```python
from build123d import *

# Parameters (mm, degrees)
F0_W     = 72.2630545497
F0_H     = 70.4785098787
F1_DEPTH = 25.4
F2_R     = 31.75
F3_DEPTH = 25.401
F5_DEPTH = 104.0980848


# Not quite as in the source:
# - an extrude ends at something that could not be found from the text; its depth is read off the source's solid


with BuildPart() as f1:
    # F0 (on Front) → F1 (new body)
    with BuildSketch(Plane.XZ):
        with Locations((36.1315272748, 34.5705245854)):
            Rectangle(F0_W, F0_H)
    extrude(amount=F1_DEPTH)

    # F2 (on face) → F3 (cut, through all)
    with BuildSketch(Plane.XZ.offset(25.4)):
        with Locations((37.1520854533, 36.7239564657)):
            Circle(F2_R)
    extrude(amount=-F3_DEPTH, mode=Mode.SUBTRACT)

    # F4 (on face) → F5 (join, through all)
    with BuildSketch(Plane.YZ.offset(72.2630545497)):
        Polygon((-12.5073632225, 25.324318558), (-5.8186161332, 49.7185699642), (-14.3406965322, 53.0769830369), (-21.9502989203, 25.324318558), align=None)
    extrude(amount=F5_DEPTH)


solid = f1.part
```
Source: CAD feature listing. Evaluate the final solid. Frame: model axes, mm. A direction names the side the tool comes from. Give positions to 0.01 mm unless a question says otherwise; leave off trailing zeros. Loops run counter-clockwise (first coordinate to the right, second up) from the corner with the lowest first, then second, coordinate; pieces in that order, holes last. Notation, with made-up numbers: (5.25, 73) - (24.25, 73) arc R33 cw to (24.25, 103) - close; hole circle Ø7 at (10, 51.5). An arc over 180 degrees is marked (long way). Use CSV: the item, a comma, the result in double quotes.
1) Cut plane C-C (y = -8). Output: boundary loops of the cut face in (x, z).
Worked out:
outline,"(0, -0.67) - (72.26, -0.67) - (72.26, 41.76) - (176.36, 41.76) - (176.36, 50.58) - (72.26, 50.58) - (72.26, 69.81) - (0, 69.81) - close; hole circle Ø63.5 at (37.15, 36.72)"
2) Pin query (flat end, axial travel): P1, Ø3, axis at x = 106, y = -13.5, coming from the +Z side; P2, Ø3, axis at x = 85.5, z = 56.5, coming from the +Y side; P3, Ø8, axis at y = -15.5, z = 17.5, coming from the +X side; P4, Ø7.5, axis at x = 103, y = -19.5, coming from the -Z side. Return the tip coordinate at first contact, or that it passes through.
Worked out:
P1,"stops at z = 53.08"
P2,"passes through"
P3,"stops at x = 72.26"
P4,"stops at z = 25.32"
3) Cut plane D-D (z = 40.5). Output: boundary loops of the cut face in (x, y), and give its area (3 significant figures).
Worked out:
outline,"(0, -25.4) - (5.63, -25.4) - (5.63, 0) - (0, 0) - close; (68.68, -25.4) - (72.26, -25.4) - (72.26, -17.79) - (176.36, -17.79) - (176.36, -8.35) - (72.26, -8.35) - (72.26, 0) - (68.68, 0) - close"
area,"1,220 mm^2"
4) Set-up query: faces 5 (the flat face through (36, 0, 4)), 6 (the flat face through (123.583, -18.092, 39.395)), 7 (the flat face through (123.58, -9.21, 37.35)). Return all of +Z, -Z, +X, -X, +Y, -Y with unobstructed straight access to the full face (end or side cutting, diameter ignored); none if empty.
Worked out:
face 5,"+Z, -Z, +X, -X, +Y"
face 6,"+Z, +X, -Y"
face 7,"-Z, +X, +Y"
5) Mould query, pull axis Z, two halves, no side actions, for faces 1 (the flat face through (124, -17, 25.324)), 2 (the cylindrical face through (67.436, -12.878, 46.261)), 3 (the flat face through (123.583, -10.02, 51.374)), 4 (the flat face through (0, -13, 34)). Classes: +Z half, -Z half, draft (parallel to the pull), parting line (faces both ways), or undercut.
Worked out:
face 1,"-Z half"
face 2,"undercut"
face 3,"+Z half"
face 4,"draft"
6) Cut plane B-B (x = 41). Output: boundary loops of the cut face in (y, z), and give its area (3 significant figures).
Worked out:
outline,"(-25.4, -0.67) - (0, -0.67) - (0, 5.21) - (-25.4, 5.21) - close; (-25.4, 68.24) - (0, 68.24) - (0, 69.81) - (-25.4, 69.81) - close"
area,"189 mm^2"
7) Line query: line 1 (X direction, y = -22.25, z = 38); line 2 (Z direction, x = 23, y = -23.25); line 3 (X direction, y = -13, z = 19). Output: solid intervals per line, ascending.
Worked out:
line 1,"x = 0 to 5.43, 68.88 to 72.26"
line 2,"z = -0.67 to 8.3, 65.15 to 69.81"
line 3,"x = 0 to 10.81, 63.49 to 72.26"
8) Cut plane A-A (z = 23). Output: boundary loops of the cut face in (x, y), and give its area (3 significant figures).
Worked out:
outline,"(0, -25.4) - (8.52, -25.4) - (8.52, 0) - (0, 0) - close; (65.78, -25.4) - (72.26, -25.4) - (72.26, 0) - (65.78, 0) - close"
area,"381 mm^2"
